Autodesk Inventor part; units mm, degrees
ref_plane "YZ Plane" through (0, 0, 0) normal (1, 0, 0) x (0, 1, 0)
ref_plane "XZ Plane" through (0, 0, 0) normal (0, 1, 0) x (-1, 0, 0)
ref_plane "XY Plane" through (0, 0, 0) normal (0, 0, 1) x (1, 0, 0)
sketch "Sketch1" plane through (0, 0, 0) normal (0, 0, 1) x (1, 0, 0)
  line L0 (-13, 20) -> (13, 20)
  line L1 (13, 20) -> (13, -20)
  line L2 (13, -20) -> (-13, -20)
  line L3 (-13, -20) -> (-13, 20)
  line L4 (18, 25) -> (-18, 25)
  line L5 (-18, 25) -> (-18, -25)
  line L6 (-18, -25) -> (18, -25)
  line L7 (18, -25) -> (18, 25)
  point P0 (0, 0)
  point P1 (-13, 0)
  point P2 (0, 20)
  dimension "d0" = 26
  dimension "d1" = 40
  dimension "d2" = 5
extrude "Extrusion1" add sketch "Sketch1" along normal blind 12.5
sketch "Sketch3" plane through (0, 0, 12.5) normal (0, 0, 1) x (1, 0, 0)
  line L0 (-2.5, -25) -> (-2.5, -20)
  line L1 (13, -20) -> (-13, -20)
  line L2 (-13, -20) -> (-13, 20)
  line L3 (-13, 20) -> (13, 20)
  line L4 (-2.5, 20) -> (-2.5, 25)
  line L5 (18, 25) -> (-18, 25)
  line L6 (-18, 25) -> (-18, -25)
  line L7 (-18, -25) -> (18, -25)
  line L8 (-18, -25) -> (18, -25)
  line L9 (18, -25) -> (18, 25)
  line L10 (18, 25) -> (-18, 25)
  line L11 (-13, 20) -> (13, 20)
  line L12 (13, 20) -> (13, -20)
  line L13 (13, -20) -> (-13, -20)
  line L14 (-13, -20) -> (-13, 20)
  line L15 (-18, 25) -> (-18, -25)
  point P0 (0, 0)
extrude "Extrusion3" add sketch "Sketch3" along normal blind 5
sketch "Sketch4" plane through (0, 0, 0) normal (0, 0, -1) x (-1, 0, 0)
  line L0 (-13, 20) -> (13, 20)
  line L1 (-18, 25) -> (18, 25)
  line L2 (-10.5, 25) -> (10.5, 25)
  line L3 (10.5, 25) -> (10.5, 20)
  line L4 (10.5, 20) -> (-10.5, 20)
  line L5 (-10.5, 20) -> (-10.5, 25)
  point P0 (0, 0)
  point P1 (0, 25)
  point P2 (0, 25)
  dimension "d11" = 21
extrude "Extrusion4" cut sketch "Sketch4" against normal blind 1
sketch "Sketch5" plane through (-18, -25, 0) normal (0, -1, 0) x (1, 0, 0)
  line L0 (0, 0) -> (36, 0)
  line L1 (17, 0) -> (19, 0)
  line L2 (19, 0) -> (19, 2)
  line L3 (19, 2) -> (17, 2)
  line L4 (17, 2) -> (17, 0)
  point P0 (18, 0)
  point P1 (18, 0)
  dimension "d15" = 2
extrude "Extrusion5" cut sketch "Sketch5" against normal up to surface (45 mm away)
pattern_linear "Rectangular Pattern1" count 7 spacing 4 along (1, 0, 0) of "Extrusion5" first direction both ways yes
sketch "Sketch6" plane through (13, -25, 0) normal (0, -1, 0) x (1, 0, 0)
  circle A0 centre (-13, 12.5) radius 2.5
  point P0 (-13, 0)
  dimension "d22" = 12.5
  dimension "d23" = 5
extrude "Extrusion6" cut sketch "Sketch6" against normal through all
sketch "Sketch7" plane through (0, 0, 0) normal (0, 0, -1) x (-1, 0, 0)
  line L0 (-13, -25) -> (-13, 20)
  line L1 (-13, 20) -> (-10.5, 20)
  line L2 (-10.5, 20) -> (-10.5, 25)
  line L3 (-18, 25) -> (-10.5, 25)
  line L4 (-18, -25) -> (-18, 25)
  line L5 (-13, -25) -> (-18, -25)
  line L6 (-18, 25) -> (-13, 25)
  line L7 (-13, 25) -> (-13, -25)
  line L8 (-13, -25) -> (-18, -25)
  line L9 (-18, -25) -> (-18, 25)
  line L10 (13, -25) -> (18, -25)
  line L11 (18, -25) -> (18, 25)
  line L12 (18, 25) -> (13, 25)
  line L13 (13, 25) -> (13, -25)
  line L14 (-18, 25) -> (-10.5, 25)
  point P0 (0, 0)
extrude "Extrusion7" add sketch "Sketch7" along normal blind 5 contours L5 L4 L3 L7 L0 | L13 L12 L11 L10
fillet "Fillet3" radius 5 4 edges at (18, 25, 6.25) (18, -25, 6.25) (-18, -25, 6.25) (-18, 25, 6.25)
sketch "Sketch8" plane through (0, 0, 17.5) normal (0, 0, 1) x (1, 0, 0)
  circle A0 centre (-9, 0) radius 3
  point P0 (0, 0)
  dimension "d31" = 6
  dimension "d34" = 9
extrude "Extrusion8" cut sketch "Sketch8" against normal blind 3
sketch "Sketch9" plane through (-9, 0, 14.5) normal (0, 0, 1) x (1, 0, 0)
  circle A0 centre (0, 0) radius 3
  circle A1 centre (0, 0) radius 1.75
  point P0 (9, 0)
  dimension "d37" = 3.5
extrude "Extrusion9" cut sketch "Sketch9" against normal through all contours A1
mirror "Mirror1" about plane through (0, 0, 0) normal (1, 0, 0) of "Extrusion8", "Extrusion9"
properties part number "wire block"
Input: part model. Units: mm. Frame: model coordinates. A direction names the side the tool comes from. Round coordinates to 2 decimals unless told otherwise and drop trailing zeros. Loops run counter-clockwise (first coordinate to the right, second up) from the corner with the lowest first, then second, coordinate; pieces in that order, holes last. Notation, with made-up numbers: (-21.5, -24.75) -> (-17.5, -24.75) arc R19 ccw to (-17.5, 8.25) -> close; hole circle Ø10 at (-17, -13). An arc over 180 degrees is marked (long way). Write each question's results on one line, items separated by ' | '.
1. Set-up query: faces 4 (the face through (11, 0, 14.5)), 5 (the face through (-7, 0, 12.5)), 6 (the face through (-12, -23, 2)). Return all of +Z, -Z, +X, -X, +Y, -Y with unobstructed straight access to the full face (end or side cutting, diameter ignored); none if empty.
Geometry results:
face 4: +Z | face 5: -Z | face 6: -Z, -Y
2. Section A-A (x = 0). Return loops of the section in (y, z), and give its area (3 significant figures).
Geometry results:
outline: (-25, 2) -> (-20, 2) -> (-20, 10) -> (-25, 10) -> close; (-25, 15) -> (25, 15) -> (25, 17.5) -> (-25, 17.5) -> close; (20, 1) -> (25, 1) -> (25, 10) -> (20, 10) -> close | area: 210 mm2
3. Section C-C (z = 6). Return loops of the section in (x, y), and give its area (3 significant figures).
Geometry results:
outline: (-18, -20) arc R5 ccw to (-13, -25) -> (13, -25) arc R5 ccw to (18, -20) -> (18, 20) arc R5 ccw to (13, 25) -> (-13, 25) arc R5 ccw to (-18, 20) -> close; hole (-13, -20) -> (13, -20) -> (13, 20) -> (-13, 20) -> close | area: 739 mm2
4. Ray query, line 1 (Y direction, x = -3.5, z = 5); line 2 (Z direction, x = 0, y = -22.5); line 3 (Y direction, x = -9, z = 16.05). Return the intervals inside material, ascending. Write a range as from..to.
Geometry results:
line 1: -25..-20, 20..25 | line 2: 2..10, 15..17.5 | line 3: -25..-3, 3..25
5. Section D-D (z = 16). Return loops of the section in (x, y).
Geometry results:
outline: (-18, -20) arc R5 ccw to (-13, -25) -> (13, -25) arc R5 ccw to (18, -20) -> (18, 20) arc R5 ccw to (13, 25) -> (-13, 25) arc R5 ccw to (-18, 20) -> close; hole circle Ø6 at (-9, 0); hole circle Ø6 at (9, 0)
6. Mould query, pull axis Y, two halves, no side actions, for faces 1 (the face through (-11, -23, 1)), 2 (the face through (0, 25, 9)), 3 (the face through (7, 0, 12.5)). Classes: +Y half, -Y half, draft (parallel to the pull), parting line (faces both ways), or undercut.
Geometry results:
face 1: draft | face 2: +Y half | face 3: undercut
7. First-contact query: P1, Ø7, axis at x = 9, y = 0, coming from the +Z side; P2, Ø1.2, axis at x = -12, y = 22.5, coming from the -Z side; P3, Ø1.6, axis at y = -22.5, z = 1, coming from the -X side; P4, Ø10, axis at x = -2, y = -2, coming from the -Z side. Flat tips, straight axial feed; report the tip coordinate or a pass-through.
Geometry results:
P1: z = 17.5 | P2: z = 0 | P3: x = -17.7 | P4: z = 12.5
8. Section B-B (y = 0). Return loops of the section in (x, z), and give its area (3 significant figures).
Geometry results:
outline: (-18, -5) -> (-13, -5) -> (-13, 12.5) -> (-10.75, 12.5) -> (-10.75, 14.5) -> (-12, 14.5) -> (-12, 17.5) -> (-18, 17.5) -> close; (-7.25, 12.5) -> (-2.5, 12.5) arc R2.5 cw to (2.5, 12.5) -> (7.25, 12.5) -> (7.25, 14.5) -> (6, 14.5) -> (6, 17.5) -> (-6, 17.5) -> (-6, 14.5) -> (-7.25, 14.5) -> close; (10.75, 12.5) -> (13, 12.5) -> (13, -5) -> (18, -5) -> (18, 17.5) -> (12, 17.5) -> (12, 14.5) -> (10.75, 14.5) -> close | area: 295 mm2
